For this review, take the finished solid that the model builds, in its own axes (mm). A direction names the side the tool comes from. Give positions to 0.01 mm unless a question says otherwise; leave off trailing zeros. Order: outer loops, then holes, each group sorted by start corner. A loop starts at its lowest first (then second) coordinate and runs counter-clockwise, first axis right, second up. Notation, with made-up numbers: (11.5, 79.25) - (24.5, 79.25) arc R20 ccw to (24.5, 90.25) - close; hole circle Ø9 at (44, 30). An arc over 180 degrees is marked (long way). Use a Markdown table: item, result. Add a question column.
1) We need section A-A on x = 0. Write out the cut boundary in (y, z), then the cut area to 3 significant figures.
2) We need section B-B on z = -3.5. Write out the cut boundary in (x, y).
3) We need section C-C on y = 0. Write out the cut boundary in (x, z).
4) Wall thickness on L1, parallel to X at y = -2.75, z = -4; L2, parallel to X at y = -0.25, z = 4.5; L3, parallel to Z at x = -0.75, y = 0: over which ranges is each line inside the solid? List them lowest first.
5) Clearance check with flat-ended pins moving along their axes: P1, Ø4, axis at x = 0, y = 2, coming from the -Z side; P2, Ø1.5, axis at x = -0.5, y = 0.5, coming from the +Z side; P3, Ø4, axis at y = -7, z = -2, coming from the +X side. State where each tip first meets the part, or that it passes through.
6) Machinability: for faces 1 (the face through (-7.493, 0.33, 6.465)), 2 (the face through (0, 0, 0)), 3 (the face through (-9, 0, -2)), 4 (the face through (-8.248, 5.287, -2.535)), which of the approach directions +Z, -Z, +X, -X, +Y, -Y give a long, thin tool a straight path to every point of the face, cutting with its end or side? Answer none if there is none.
7) Mouldability with a two-part tool opening along Y and no side actions: class faces 5 (the face through (8.287, -5.248, -2.535)), 6 (the face through (0, -4.2, -3)), 7 (the face through (8.287, 5.248, -2.535)), 8 (the face through (-2.222, -10.006, 1.972)) as released by +Y, released by -Y, zero draft, split by the parting line, or undercut.
8) We need section D-D on z = 5.5. Write out the cut boundary in (x, y).
```python
from build123d import *

# Parameters (mm, degrees)
F0_R         = 10.25
F1_DEPTH     = 4
F2_W         = 18
F2_H         = 12
F3_DEPTH     = 5
F4_W         = 15.4
F4_H         = 8.4
F5_DEPTH     = 5
F6_R         = 7.5
F7_DEPTH     = 5
F9_DEPTH     = 5
F10_T1_DEPTH = 11.25


# Not quite as in the source:
# - a fillet or chamfer that OpenCascade refuses, or shapes differently, is made with other operations: its cross-section is extruded or revolved along the edge and cut away or added


with BuildPart() as f1:
    # F0 (on Top) → F1 (new body)
    with BuildSketch(Plane.XY):
        Circle(F0_R)
    extrude(amount=F1_DEPTH)

    # F2 (on face) → F3 (join)
    with BuildSketch(Plane(origin=(0, 0, 0), x_dir=(1, 0, 0), z_dir=(0, 0, -1))):
        Rectangle(F2_W, F2_H)
    extrude(amount=F3_DEPTH)

    # F4 (on face) → F5 (cut)
    with BuildSketch(Plane(origin=(0, 0, -5), x_dir=(1, 0, 0), z_dir=(0, 0, -1))):
        Rectangle(F4_W, F4_H)
    extrude(amount=-F5_DEPTH, mode=Mode.SUBTRACT)

    # F6 (on face) → F7 (join)
    with BuildSketch(Plane.XY.offset(4)):
        Circle(F6_R)
    extrude(amount=F7_DEPTH)

    # F8 (on face) → F9 (cut)
    with BuildSketch(Plane.XY.offset(9)):
        with BuildLine():
            ThreePointArc((3.1, 4.25), (0, 5.2604657588), (-3.1, 4.25))
            Line((-3.1, 4.25), (-3.1, -4.25))
            ThreePointArc((-3.1, -4.25), (0, -5.2604657588), (3.1, -4.25))
            Line((3.1, -4.25), (3.1, 4.25))
        make_face()
    extrude(amount=-F9_DEPTH, mode=Mode.SUBTRACT)

    # F10: fillet of radius 2.5 on 4 edges, made by hand

    # F10_s2 → F10_t1 (cut)
    with BuildSketch(Plane.XY.offset(-11.25)):
        with BuildLine():
            ThreePointArc((-6.5, 6), (-8.267766953, 5.267766953), (-9, 3.5))
            Line((-9, 3.5), (-9, 6))
            Line((-9, 6), (-6.5, 6))
        make_face()
        with BuildLine():
            ThreePointArc((-9, -3.5), (-8.267766953, -5.267766953), (-6.5, -6))
            Line((-6.5, -6), (-9, -6))
            Line((-9, -6), (-9, -3.5))
        make_face()
        with BuildLine():
            ThreePointArc((9, -3.5), (8.267766953, -5.267766953), (6.5, -6))
            Line((6.5, -6), (9, -6))
            Line((9, -6), (9, -3.5))
        make_face()
        with BuildLine():
            ThreePointArc((9, 3.5), (8.267766953, 5.267766953), (6.5, 6))
            Line((6.5, 6), (9, 6))
            Line((9, 6), (9, 3.5))
        make_face()
    extrude(amount=F10_T1_DEPTH, mode=Mode.SUBTRACT)


solid = f1.part
```
Checked values:
| question | item | result |
|---|---|---|
| 1 | outline | (-10.25, 0) - (-6, 0) - (-6, -5) - (-4.2, -5) - (-4.2, 0) - (4.2, 0) - (4.2, -5) - (6, -5) - (6, 0) - (10.25, 0) - (10.25, 4) - (7.5, 4) - (7.5, 9) - (5.26, 9) - (5.26, 4) - (-5.26, 4) - (-5.26, 9) - (-7.5, 9) - (-7.5, 4) - (-10.25, 4) - close |
| 1 | area | 122 mm² |
| 2 | outline | (-9, -3.5) arc R2.5 ccw to (-6.5, -6) - (6.5, -6) arc R2.5 ccw to (9, -3.5) - (9, 3.5) arc R2.5 ccw to (6.5, 6) - (-6.5, 6) arc R2.5 ccw to (-9, 3.5) - close; hole (-7.7, -4.2) - (7.7, -4.2) - (7.7, 4.2) - (-7.7, 4.2) - close |
| 3 | outline | (-10.25, 0) - (-9, 0) - (-9, -5) - (-7.7, -5) - (-7.7, 0) - (7.7, 0) - (7.7, -5) - (9, -5) - (9, 0) - (10.25, 0) - (10.25, 4) - (7.5, 4) - (7.5, 9) - (3.1, 9) - (3.1, 4) - (-3.1, 4) - (-3.1, 9) - (-7.5, 9) - (-7.5, 4) - (-10.25, 4) - close |
| 4 | L1 | -9 to -7.7, 7.7 to 9 |
| 4 | L2 | -7.5 to -3.1, 3.1 to 7.5 |
| 4 | L3 | 0 to 4 |
| 5 | P1 | z = 0 |
| 5 | P2 | z = 4 |
| 5 | P3 | x = 8.5 |
| 6 | face 1 | +Z |
| 6 | face 2 | -Z |
| 6 | face 3 | -Z, -X, +Y, -Y |
| 6 | face 4 | -Z, -X, +Y |
| 7 | face 5 | released by -Y |
| 7 | face 6 | undercut |
| 7 | face 7 | released by +Y |
| 7 | face 8 | split by the parting line |
| 8 | outline | circle Ø15 at (0, 0); hole (-3.1, -4.25) arc R5.26 ccw to (3.1, -4.25) - (3.1, 4.25) arc R5.26 ccw to (-3.1, 4.25) - close |
